Geometry check sheet. Reference: the model listing, model coordinates, mm. Face numbers are marked on the shaded views. A direction names the side the tool comes from. Coordinates: 2 decimals unless noted, no trailing zeros. Loops run counter-clockwise (first coordinate to the right, second up) from the corner with the lowest first, then second, coordinate; pieces in that order, holes last.
from build123d import *

# Parameters (mm, degrees)
F0_R     = 11.2903
F1_DEPTH = 6.35


with BuildPart() as f1:
    # F0 (on Top) → F1 (new body)
    with BuildSketch(Plane.XY):
        with BuildLine():
            ThreePointArc((-11.346624, 37.154203), (-11.72432, 25.907716), (-9.469638, 14.883083))
            ThreePointArc((-9.469638, 14.883083), (-15.276948, 8.82015), (-17.623946, 0.759406))
            ThreePointArc((-17.623946, 0.759406), (-28.2989, -2.800299), (-37.849796, -8.750637))
            ThreePointArc((-37.849796, -8.750637), (-45.082615, -15.032073), (-45.168132, -24.611364))
            Line((-45.168132, -24.611364), (-41.839084, -22.689337))
            ThreePointArc((-41.839084, -22.689337), (-35.905842, -12.195564), (-26.647972, -19.916605))
            ThreePointArc((-26.647972, -19.916605), (-31.856515, -27.307858), (-40.569084, -24.889041))
            Line((-40.569084, -24.889041), (-43.898132, -26.811068))
            ThreePointArc((-43.898132, -26.811068), (-35.559465, -31.526653), (-26.503172, -28.403566))
            ThreePointArc((-26.503172, -28.403566), (-16.57458, -23.107417), (-8.154309, -15.642488))
            ThreePointArc((-8.154309, -15.642488), (0, -17.6403), (8.154309, -15.642488))
            ThreePointArc((8.154309, -15.642488), (16.57458, -23.107417), (26.503172, -28.403566))
            ThreePointArc((26.503172, -28.403566), (35.559465, -31.526653), (43.898132, -26.811068))
            Line((43.898132, -26.811068), (40.569084, -24.889041))
            ThreePointArc((40.569084, -24.889041), (27.105319, -17.276548), (42.345172, -19.916605))
            ThreePointArc((42.345172, -19.916605), (42.217614, -21.325875), (41.839084, -22.689337))
            Line((41.839084, -22.689337), (45.168132, -24.611364))
            ThreePointArc((45.168132, -24.611364), (45.082615, -15.032073), (37.849796, -8.750637))
            ThreePointArc((37.849796, -8.750637), (28.2989, -2.800299), (17.623946, 0.759406))
            ThreePointArc((17.623946, 0.759406), (15.276948, 8.82015), (9.469638, 14.883083))
            ThreePointArc((9.469638, 14.883083), (11.72432, 25.907716), (11.346624, 37.154203))
            ThreePointArc((11.346624, 37.154203), (9.52315, 46.558727), (1.27, 51.422432))
            Line((1.27, 51.422432), (1.27, 47.578378))
            ThreePointArc((1.27, 47.578378), (5.981983, 44.914195), (7.8486, 39.83321))
            ThreePointArc((7.8486, 39.83321), (-5.080984, 33.851227), (-1.27, 47.578378))
            Line((-1.27, 47.578378), (-1.27, 51.422432))
            ThreePointArc((-1.27, 51.422432), (-9.52315, 46.558727), (-11.346624, 37.154203))
        make_face()
        with BuildLine():
            ThreePointArc((-13.175642, -11.729563), (-17.713182, -16.022689), (-22.842613, -19.587676))
            ThreePointArc((-22.842613, -19.587676), (-24.399928, -14.087305), (-28.384732, -9.988445))
            ThreePointArc((-28.384732, -9.988445), (-22.732647, -7.328721), (-16.745921, -5.545659))
            ThreePointArc((-16.745921, -5.545659), (-15.276948, -8.82015), (-13.175642, -11.729563))
        make_face(mode=Mode.SUBTRACT)
        with BuildLine():
            ThreePointArc((16.745921, -5.545659), (22.732647, -7.328721), (28.384732, -9.988445))
            ThreePointArc((28.384732, -9.988445), (24.399928, -14.087305), (22.842613, -19.587676))
            ThreePointArc((22.842613, -19.587676), (17.713182, -16.022689), (13.175642, -11.729563))
            ThreePointArc((13.175642, -11.729563), (15.276948, -8.82015), (16.745921, -5.545659))
        make_face(mode=Mode.SUBTRACT)
        Circle(F0_R, mode=Mode.SUBTRACT)
        with BuildLine():
            ThreePointArc((-3.570279, 17.275222), (-5.019465, 23.35141), (-5.542119, 29.576122))
            ThreePointArc((-5.542119, 29.576122), (0, 28.17461), (5.542119, 29.576122))
            ThreePointArc((5.542119, 29.576122), (5.019465, 23.35141), (3.570279, 17.275222))
            ThreePointArc((3.570279, 17.275222), (0, 17.6403), (-3.570279, 17.275222))
        make_face(mode=Mode.SUBTRACT)
        with BuildLine():
            ThreePointArc((-26.647972, -19.916605), (-35.905842, -12.195564), (-41.839084, -22.689337))
            ThreePointArc((-41.839084, -22.689337), (-41.293659, -23.840905), (-40.569084, -24.889041))
            ThreePointArc((-40.569084, -24.889041), (-31.856515, -27.307858), (-26.647972, -19.916605))
        make_face()
        with BuildLine():
            ThreePointArc((1.27, 47.578378), (0, 47.68181), (-1.27, 47.578378))
            ThreePointArc((-1.27, 47.578378), (-5.080984, 33.851227), (7.8486, 39.83321))
            ThreePointArc((7.8486, 39.83321), (5.981983, 44.914195), (1.27, 47.578378))
        make_face()
        with BuildLine():
            ThreePointArc((40.569084, -24.889041), (41.293659, -23.840905), (41.839084, -22.689337))
            ThreePointArc((41.839084, -22.689337), (42.217614, -21.325875), (42.345172, -19.916605))
            ThreePointArc((42.345172, -19.916605), (27.105319, -17.276548), (40.569084, -24.889041))
        make_face()
    extrude(amount=F1_DEPTH)


solid = f1.part
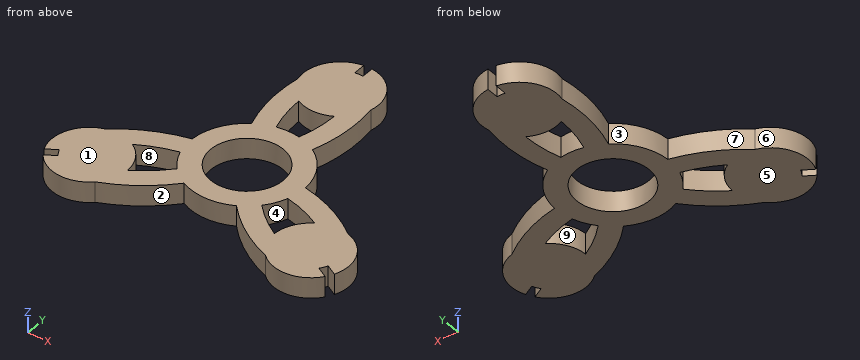
(1) Sectioned sample at D-D on x = 33. Record the cut outline in (y, z), and give its area (3 significant figures).
Findings:
outline: (-31.48, 0) - (-5.34, 0) - (-5.34, 6.35) - (-31.48, 6.35) - close
area: 166 mm2
(2) Sectioned sample at C-C on y = 41.5. Record the cut outline in (x, z), and give its area (3 significant figures).
Findings:
outline: (-11.54, 0) - (11.54, 0) - (11.54, 6.35) - (-11.54, 6.35) - close
area: 147 mm2
(3) Scan lines: L1, parallel to X at y = -16, z = 6.25; L2, parallel to Y at x = -1.5, z = 0.75; L3, parallel to Y at x = -13.5, z = 1.5. Record each from-to range of solid material in increasing order.
Findings:
L1: x = -45.48 to -23.52, -17.69 to -8.48, -7.43 to 7.43, 8.48 to 17.69, 23.52 to 45.48
L2: y = -17.58 to -11.19, 11.19 to 17.58, 28.27 to 51.39
L3: y = -20.78 to -12.08, -11.35 to 11.35
(4) Sectioned sample at A-A on x = 0. Record the cut outline in (y, z).
Findings:
outline: (-17.64, 0) - (-11.29, 0) - (-11.29, 6.35) - (-17.64, 6.35) - close; (11.29, 0) - (17.64, 0) - (17.64, 6.35) - (11.29, 6.35) - close; (28.17, 0) - (47.68, 0) - (47.68, 6.35) - (28.17, 6.35) - close
(5) Draft check along Y on the marked faces 6, 7, 8 and 9. Enter one of: +Y half, -Y half, draft (parallel to the pull), parting line (faces both ways), or undercut.
Findings:
face 6: parting line
face 7: +Y half
face 8: undercut
face 9: undercut
(6) Access from +Z, -Z, +X, -X, +Y, -Y to the whole of each face (thin tool, end or side, straight path). Record for the marked faces 1, 2, 3, 4 and 5.
Findings:
face 1: +Z, +X, -X, +Y, -Y
face 2: +Z, -Z, -Y
face 3: +Z, -Z, -X
face 4: +Z, -Z
face 5: -Z, +X, -X, +Y, -Y
(7) Gauge pin test, flat ends, axial feed: pin 1 Ø1 at (x, y) = (-26.5, -4.5) entering from -Z; pin 2 Ø2 at (x, z) = (5.5, 4.5) entering from +Y; pin 3 Ø2 at (x, z) = (-12.5, 1.5) entering from -Y; pin 4 Ø1.2 at (y, z) = (50, 4.5) entering from +X. Record the tip position at first contact, or that the pin passes through.
Findings:
pin 1: stops at z = 0
pin 2: stops at y = 50.59
pin 3: stops at y = -20.78
pin 4: stops at x = 6.66
(8) Sectioned sample at B-B on y = -4. Record the cut outline in (x, z), and give its area (3 significant figures).
Findings:
outline: (-30.68, 0) - (-10.56, 0) - (-10.56, 6.35) - (-30.68, 6.35) - close; (10.56, 0) - (30.68, 0) - (30.68, 6.35) - (10.56, 6.35) - close
area: 256 mm2
